from build123d import *

# Parameters (mm, degrees)
F0_W     = 142.05
F0_H     = 90
F1_DEPTH = 12
F2_W     = 24
F2_H     = 20
F3_DEPTH = 12
F4_DEPTH = 10.02627
F5_W     = 142.05
F5_H     = 1.43163
F6_DEPTH = 25


with BuildPart() as f1:
    # F0 (on Front) → F1 (new body)
    with BuildSketch(Plane.XZ):
        with Locations((71.025, 45)):
            Rectangle(F0_W, F0_H)
    extrude(amount=F1_DEPTH)

    # F2 (on face) → F3 (join)
    with BuildSketch(Plane.XZ.offset(12)):
        with Locations((0, 45)):
            Rectangle(F2_W, F2_H)
        with Locations((142.05, 45)):
            Rectangle(F2_W, F2_H)
    extrude(amount=-F3_DEPTH)

    # F4 (cut): a face of the model
    f4_faces = [f1.faces().sort_by_distance(p)[0] for p in [
        (71.025, -6, 90),
    ]]
    extrude(f4_faces, amount=-F4_DEPTH, mode=Mode.SUBTRACT)

    # F5 (on face) → F6 (cut)
    with BuildSketch(Plane.XZ.offset(12)):
        with Locations((71.025, 79.257915)):
            Rectangle(F5_W, F5_H)
    extrude(amount=-F6_DEPTH, mode=Mode.SUBTRACT)


solid = f1.part
Geometry check sheet. Reference: the model listing, model coordinates, mm. A direction names the side the tool comes from. Round coordinates to 2 decimals unless told otherwise and drop trailing zeros. Order: outer loops, then holes, each group sorted by start corner. A loop starts at its lowest first (then second) coordinate and runs counter-clockwise, first axis right, second up. Notation, with made-up numbers: M -36.75,31 L 13.25,31 A31 cw 13.25,60 Z; hole C 74,-17.5 d10. An arc over 180 degrees is marked long. Write each question's results on one line, items separated by ' | '. Start each with the question number.
1. Cross-section at B-B on z = 56.5. Record the boundary of the cut face in (x, y).
2. Go/stop test with flat-tipped pins: P1, Ø6, axis at x = -9, y = -8.5, coming from the -Z side; P2, Ø1.5, axis at y = -3, z = 56.5, coming from the +X side; P3, Ø6, axis at x = -4.5, y = -4, coming from the +Z side. Record where each tip stops, or that it passes through.
3. Material ranges on L1, parallel to X at y = -5, z = 75.5, recorded low to high. Write a range as from..to.
4. Cross-section at A-A on y = -8. Record the boundary of the cut face in (x, z).
5. Set-up check for faces 1 (the face through (0, -6, 17)), 2 (the face through (0, -6, 67)), 3 (the face through (148, -6, 55)), 4 (the face through (142.05, -6, 17)): record each of +Z, -Z, +X, -X, +Y, -Y from which the full face is reachable in a straight line by a thin tool's end or side.
Resolved:
1) outline: M 0,-12 L 142.05,-12 L 142.05,0 L 0,0 Z
2) P1: z = 35 | P2: x = 142.05 | P3: z = 55
3) L1: 0..142.05
4) outline: M -12,35 L 0,35 L 0,0 L 142.05,0 L 142.05,35 L 154.05,35 L 154.05,55 L 142.05,55 L 142.05,78.54 L 0,78.54 L 0,55 L -12,55 Z
5) face 1: -Z, -X, +Y, -Y | face 2: +Z, -X, +Y, -Y | face 3: +Z, +X, +Y, -Y | face 4: -Z, +X, +Y, -Y
